from build123d import *

# Parameters (mm, degrees)
SKETCH1_R           = 7
BOSS_EXTRUDE3_DEPTH = 10
SKETCH4_R           = 4.05
CUT_EXTRUDE1_DEPTH  = 4
SKETCH5_W           = 6.2
SKETCH5_H           = 4.2
CUT_EXTRUDE2_DEPTH  = 6
CUT_EXTRUDE3_DEPTH  = 4
CUT_EXTRUDE4_DEPTH  = 15.071247279
CHAMFER1_SIZE       = 2
CHAMFER1_SIZE_2     = 3.464101615
CUT_EXTRUDE5_DEPTH  = 4
FILLET1_R           = 4


with BuildPart() as part:
    # Sketch1 → Boss-Extrude3 (new body)
    with BuildSketch(Plane(origin=(0, 0, 0), x_dir=(1, 0, 0), z_dir=(0, 1, 0))):
        with Locations(Location((0, 0, 0), (0, 0, 270))):
            Circle(SKETCH1_R)
    extrude(amount=BOSS_EXTRUDE3_DEPTH)

    # Sketch4 → Cut-Extrude1 (cut)
    with BuildSketch(Plane(origin=(0, 10, 0), x_dir=(1, 0, 0), z_dir=(0, 1, 0))):
        with Locations(Location((0, 0, 0), (0, 0, 270))):
            Circle(SKETCH4_R)
    extrude(amount=-CUT_EXTRUDE1_DEPTH, mode=Mode.SUBTRACT)

    # Sketch5 → Cut-Extrude2 (cut)
    with BuildSketch(Plane.XZ):
        Rectangle(SKETCH5_W, SKETCH5_H)
    extrude(amount=-CUT_EXTRUDE2_DEPTH, mode=Mode.SUBTRACT)

    # Sketch6 → Cut-Extrude3 (cut)
    with BuildSketch(Plane.XZ):
        with BuildLine():
            ThreePointArc((0, -7), (7, 0), (0, 7))
            ThreePointArc((0, 7), (3.67817462, 0), (0, -7))
        make_face()
    extrude(amount=-CUT_EXTRUDE3_DEPTH, mode=Mode.SUBTRACT)

    # Sketch7 → Cut-Extrude4 (cut, through all)
    with BuildSketch(Plane(origin=(0, 10, 0), x_dir=(1, 0, 0), z_dir=(0, 1, 0))):
        with BuildLine():
            Line((-5, -4.898979486), (5, -4.898979486))
            ThreePointArc((5, -4.898979486), (0, -7), (-5, -4.898979486))
        make_face()
        with BuildLine():
            Line((5, 4.898979486), (-5, 4.898979486))
            ThreePointArc((-5, 4.898979486), (0, 16.797958971), (5, 4.898979486))
        make_face()
    extrude(amount=-CUT_EXTRUDE4_DEPTH, mode=Mode.SUBTRACT)

    # Chamfer1
    # the kernel refuses this chamfer: 3.464101615, 2 mm, written as the material it takes off along each edge
    with BuildSketch(Plane(origin=(0, 4, 0), x_dir=(-0.4663618278566538, 0, -0.8845940569087047), z_dir=(-0.8845940569087047, 0, 0.4663618278566538))) as chamfer1_piece_1_section:
        Polygon((7, -CHAMFER1_SIZE), (7 - CHAMFER1_SIZE_2, 0), (7, 0), align=None)
    chamfer1_piece_1 = revolve(axis=Axis((0, 4, 0), (0, -1, 0)), revolution_arc=235.596785732, mode=Mode.PRIVATE)
    chamfer1_piece_1 = chamfer1_piece_1 - Plane(origin=(-4.82182538, 5.041782237, 0), x_dir=(0.5672735741760563, 0, 0.8235294117647058), z_dir=(0, -1, 0)) * Cylinder(8.5, 29, mode=Mode.PRIVATE)
    add(chamfer1_piece_1, mode=Mode.SUBTRACT)

    # Sketch10 → Cut-Extrude5 (cut)
    with BuildSketch(Plane.XZ):
        with BuildLine():
            Line((1.820847698, -4.898979486), (1.820847698, 4.898979486))
            Line((1.820847698, 4.898979486), (2.124396614, 4.898979486))
            ThreePointArc((2.124396614, 4.898979486), (3.67817462, 0), (2.124396614, -4.898979486))
            Line((2.124396614, -4.898979486), (1.820847698, -4.898979486))
        make_face()
    extrude(amount=-CUT_EXTRUDE5_DEPTH, mode=Mode.SUBTRACT)

    # Fillet1
    # the kernel refuses this fillet: 4 mm, written as the material it takes off along each edge
    with BuildSketch(Plane(origin=(1.820847698, -9.538589297, 4.898979486), x_dir=(-1, 0, 0), z_dir=(0, 1, 0))) as fillet1_piece_1:
        with BuildLine():
            CenterArc((3.815435719, -4), FILLET1_R, 90, 72.527072621)
            Line((0, -2.798979486), (0, 0))
            Line((0, 0), (3.815435719, 0))
        make_face()
    extrude(amount=13.538589297, mode=Mode.SUBTRACT)
    with BuildSketch(Plane(origin=(1.820847698, -9.538589297, -4.898979486), x_dir=(-1, 0, 0), z_dir=(0, 1, 0))) as fillet1_piece_2:
        with BuildLine():
            CenterArc((3.815435719, 4), FILLET1_R, 197.472927379, 72.527072621)
            Line((0, 2.798979486), (0, 0))
            Line((0, 0), (3.815435719, 0))
        make_face()
    extrude(amount=13.538589297, mode=Mode.SUBTRACT)


solid = part.part
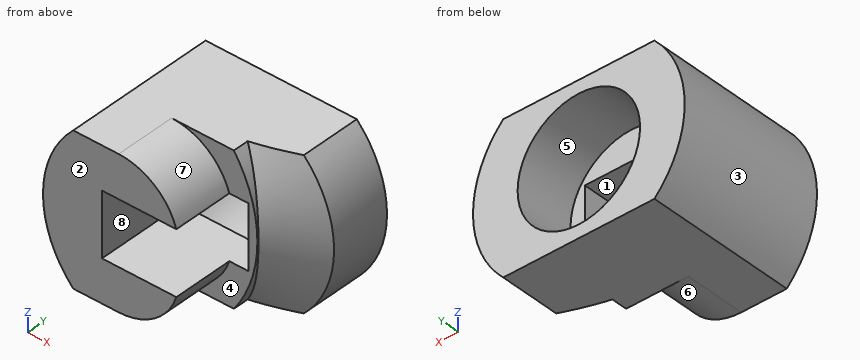
Verification items for the finished model (mm, model axes). Face numbers are marked on the shaded views. A direction names the side the tool comes from. Coordinates: 2 decimals unless noted, no trailing zeros. Order: outer loops, then holes, each group sorted by start corner. A loop starts at its lowest first (then second) coordinate and runs counter-clockwise, first axis right, second up. Notation, with made-up numbers: (17.5, 88.5) -> (54.5, 88.5) arc R22 ccw to (54.5, 107.5) -> close; hole circle Ø10 at (-3, 10.5). An arc over 180 degrees is marked (long way). Put each result on its own line as item: value. Start each with the question number.
1. Material ranges on L1, parallel to Z at x = 1, y = 5; L2, parallel to X at y = 5.25, z = -1.25; L3, parallel to X at y = 8.75, z = -3.25, recorded low to high. Write a range as [from, to].
2. Go/stop test with flat-tipped pins: pin 1 Ø1.8 at (x, y) = (0.5, 2.5) entering from -Z; pin 2 Ø3 at (y, z) = (4, -2) entering from -X; pin 3 Ø1.5 at (x, z) = (4, -3) entering from -Y. Record where each tip stops, or that it passes through.
3. Cross-section at D-D, the plane y = 1.5. Record the boundary of the cut face in (x, z).
4. Access from +Z, -Z, +X, -X, +Y, -Y to the whole of each face (thin tool, end or side, straight path). Record for the marked faces 4, 5, 6, 7 and 8.
5. Cross-section at B-B, the plane y = 7.25. Record the boundary of the cut face in (x, z).
6. Cross-section at A-A, the plane z = 0. Record the boundary of the cut face in (x, y).
7. Mould release check, pull along Z, two halves, no side actions. Record for the marked faces 1, 2 and 3: released by +Z, released by -Z, zero draft, split by the parting line, or undercut.
Computed:
1. L1: [-4.9, -2.1], [2.1, 4.9]
1. L2: [-6.89, -3.1], [3.1, 5.56]
1. L3: [-6.2, -2.42], [2.42, 6.2]
2. pin 1: z = -4.57
2. pin 2: x = -6.98
2. pin 3: y = 4.41
3. outline: (-5, -4.9) -> (-1.99, -4.9) arc R4 ccw to (1.82, -2.1) -> (-3.1, -2.1) -> (-3.1, 2.1) -> (1.82, 2.1) arc R4 ccw to (-1.99, 4.9) -> (-5, 4.9) arc R7 ccw to start
4. face 4: +X, -Y
4. face 5: +Y
4. face 6: -Z, +X, -Y
4. face 7: +Z, +X, -Y
4. face 8: +Y, -Y
5. outline: (-5, -4.9) -> (5, -4.9) arc R7 ccw to (5, 4.9) -> (-5, 4.9) arc R7 ccw to start; hole circle Ø8.1 at (0, 0)
6. outline: (-7, 0) -> (-3.1, 0) -> (-3.1, 6) -> (-4.05, 6) -> (-4.05, 10) -> (-7, 10) -> close; (3.1, 4) -> (3.68, 4) -> (3.68, 4.08) -> (7, 6) -> (7, 10) -> (4.05, 10) -> (4.05, 6) -> (3.1, 6) -> close
7. face 1: undercut
7. face 2: zero draft
7. face 3: split by the parting line
